from build123d import *

# Parameters (mm, degrees)
SKETCH_1_W          = 29
SKETCH_1_H          = 18
SKETCH_1_R          = 5.5
SKETCH_1_R_2        = 1.5
EXTRUDE_1_DEPTH     = 6
EXTRUDE_2_DEPTH     = 3
SKETCH_2_W          = 3
SKETCH_2_H          = 6
EXTRUDE_3_DEPTH     = 6
SKETCH_4_R          = 1.5
CUT_EXTRUDE_1_DEPTH = 6
SKETCH_5_W          = 3
SKETCH_5_H          = 6
EXTRUDE_4_DEPTH     = 6
SKETCH_7_R          = 1.5
CUT_EXTRUDE_2_DEPTH = 6
FILLET_1_R          = 2
FILLET_3_R          = 1


with BuildPart() as part:
    # Sketch 1 → Extrude 1 (new body)
    with BuildSketch(Plane(origin=(0, 0, 0), x_dir=(1, 0, 0), z_dir=(0, 1, 0))):
        with Locations((15.4, 42.3)):
            Rectangle(SKETCH_1_W, SKETCH_1_H)
        with Locations(Location((15.4, 42.3, 0), (0, 0, 270))):
            Circle(SKETCH_1_R, mode=Mode.SUBTRACT)
        with Locations(Location((6.45, 42.3, 0), (0, 0, 270))):
            Circle(SKETCH_1_R_2, mode=Mode.SUBTRACT)
        with Locations(Location((24.35, 42.3, 0), (0, 0, 270))):
            Circle(SKETCH_1_R_2, mode=Mode.SUBTRACT)
    extrude(amount=EXTRUDE_1_DEPTH)

    # Sketch 1_6 → Extrude 2 (add)
    with BuildSketch(Plane(origin=(0, 0, 0), x_dir=(1, 0, 0), z_dir=(0, 1, 0))):
        with BuildLine():
            ThreePointArc((15.4, 36.8), (19.289087297, 38.410912703), (20.9, 42.3))
            Line((20.9, 42.3), (19.3, 42.3))
            ThreePointArc((19.3, 42.3), (18.157716447, 39.542283553), (15.4, 38.4))
            Line((15.4, 38.4), (15.4, 36.8))
        make_face()
        with BuildLine():
            Line((19.3, 42.3), (20.9, 42.3))
            ThreePointArc((20.9, 42.3), (19.289087297, 46.189087297), (15.4, 47.8))
            Line((15.4, 47.8), (15.4, 46.2))
            ThreePointArc((15.4, 46.2), (18.157716447, 45.057716447), (19.3, 42.3))
        make_face()
        with BuildLine():
            ThreePointArc((9.9, 42.3), (11.510912703, 38.410912703), (15.4, 36.8))
            Line((15.4, 36.8), (15.4, 38.4))
            ThreePointArc((15.4, 38.4), (12.642283553, 39.542283553), (11.5, 42.3))
            Line((11.5, 42.3), (9.9, 42.3))
        make_face()
        with BuildLine():
            Line((15.4, 46.2), (15.4, 47.8))
            ThreePointArc((15.4, 47.8), (11.510912703, 46.189087297), (9.9, 42.3))
            Line((9.9, 42.3), (11.5, 42.3))
            ThreePointArc((11.5, 42.3), (12.642283553, 45.057716447), (15.4, 46.2))
        make_face()
    extrude(amount=EXTRUDE_2_DEPTH)

    # Sketch 2 → Extrude 3 (add)
    with BuildSketch(Plane.ZY.offset(-0.9)):
        with Locations((-46.8, 3)):
            Rectangle(SKETCH_2_W, SKETCH_2_H)
    extrude(amount=EXTRUDE_3_DEPTH)

    # Sketch 4 → Cut-Extrude 1 (cut)
    with BuildSketch(Plane.XY.offset(-45.3)):
        with Locations((-2.1, 3)):
            Circle(SKETCH_4_R)
    extrude(amount=-CUT_EXTRUDE_1_DEPTH, mode=Mode.SUBTRACT)

    # Sketch 5 → Extrude 4 (add)
    with BuildSketch(Plane(origin=(29.9, 0, 0), x_dir=(0, 0, -1), z_dir=(1, 0, 0))):
        with Locations((46.8, 3)):
            Rectangle(SKETCH_5_W, SKETCH_5_H)
    extrude(amount=EXTRUDE_4_DEPTH)

    # Sketch 7 → Cut-Extrude 2 (cut)
    with BuildSketch(Plane(origin=(0, 0, -48.3), x_dir=(-1, 0, 0), z_dir=(0, 0, -1))):
        with Locations((-32.9, 3)):
            Circle(SKETCH_7_R)
    extrude(amount=-CUT_EXTRUDE_2_DEPTH, mode=Mode.SUBTRACT)

    # Fillet 1
    fillet_1_edges = [part.edges().sort_by_distance(p)[0] for p in [
        (29.9, 3, -33.3),
        (0.9, 3, -33.3),
        (0.9, 3, -51.3),
        (29.9, 3, -51.3),
    ]]
    fillet(fillet_1_edges, radius=FILLET_1_R)

    # Fillet 3
    fillet_3_edges = [part.edges().sort_by_distance(p)[0] for p in [
        (-5.1, 0, -46.8),
        (-5.1, 6, -46.8),
        (35.9, 6, -46.8),
        (35.9, 0, -46.8),
    ]]
    fillet(fillet_3_edges, radius=FILLET_3_R)


solid = part.part
The listing builds one solid part. Answer for the finished solid, in the listing's coordinates (mm). A direction names the side the tool comes from. Give positions to 0.01 mm unless a question says otherwise; leave off trailing zeros. Loops run counter-clockwise (first coordinate to the right, second up) from the corner with the lowest first, then second, coordinate; pieces in that order, holes last. Notation, with made-up numbers: (-14.5, 11.5) - (16.5, 11.5) arc R17 ccw to (16.5, 37.5) - close; hole circle Ø4 at (65, 87.5). An arc over 180 degrees is marked (long way). Use one line per item in the form item = value.
1. Section B-B on y = 2.35 is taken. Give the vertices of the cut face in (x, z), then the cut area to 3 significant figures.
Calculated:
outline = (-5.1, -48.3) - (-3.45, -48.3) - (-3.45, -45.3) - (-5.1, -45.3) - close; (-0.75, -48.3) - (0.9, -48.3) - (0.9, -49.3) arc R2 ccw to (2.9, -51.3) - (27.9, -51.3) arc R2 ccw to (29.9, -49.3) - (29.9, -48.3) - (31.55, -48.3) - (31.55, -45.3) - (29.9, -45.3) - (29.9, -35.3) arc R2 ccw to (27.9, -33.3) - (2.9, -33.3) arc R2 ccw to (0.9, -35.3) - (0.9, -45.3) - (-0.75, -45.3) - close; (34.25, -48.3) - (35.9, -48.3) - (35.9, -45.3) - (34.25, -45.3) - close; hole circle Ø3 at (6.45, -42.3); hole circle Ø7.8 at (15.4, -42.3); hole circle Ø3 at (24.35, -42.3)
area = 476 mm^2
2. Which of the six approach directions +Z, -Z, +X, -X, +Y, -Y give full straight-line access (tool end or side, diameter ignored) to faces 5 (the face through (29.9, 3, -49)), 6 (the face through (-0.7, 1.6, -45.3)), 7 (the face through (29.9, 3, -40))?
Calculated:
face_5 = -Z, +X, +Y, -Y
face_6 = +Z, -X, +Y, -Y
face_7 = +Z, +X, +Y, -Y
3. Section C-C on z = -40 is taken. Give the vertices of the cut face in (x, y), then the cut area to 3 significant figures.
Calculated:
outline = (0.9, 0) - (12.25, 0) - (12.25, 3) - (10.4, 3) - (10.4, 6) - (0.9, 6) - close; (18.55, 0) - (29.9, 0) - (29.9, 6) - (20.4, 6) - (20.4, 3) - (18.55, 3) - close
area = 125 mm^2
4. Section D-D on x = 6.45 is taken. Give the vertices of the cut face in (y, z), then the cut area to 3 significant figures.
Calculated:
outline = (0, -51.3) - (6, -51.3) - (6, -43.8) - (0, -43.8) - close; (0, -40.8) - (6, -40.8) - (6, -33.3) - (0, -33.3) - close
area = 90.0 mm^2
5. Given pin 1 Ø0.8 at (y, z) = (2, -49) entering from -X; pin 2 Ø3 at (y, z) = (3.5, -39) entering from +X; pin 3 Ø9 at (x, z) = (15.4, -42.3) entering from +Y, each flat-ended and moving along its own axis, determine where each tip first touches the part or whether it passes through.
Calculated:
pin_1 = 0.9
pin_2 = 29.9
pin_3 = 3
6. The mould has two halves that part along Z. Classify faces 1 (the face through (31.5, 1.6, -48.3)), 2 (the face through (35.599, 0.285, -46.821)), 3 (the face through (13.29, 4.48, -37.22)), 4 (the face through (29.3, 3.04, -33.87)): pulls with the +Z half, pulls with the -Z half, needs draft (parallel to the pull), parting line crosses it, or undercut.
Calculated:
face_1 = pulls with the -Z half
face_2 = needs draft
face_3 = undercut
face_4 = pulls with the +Z half
7. Section A-A on x = 32.9 is taken. Give the vertices of the cut face in (y, z), then the cut area to 3 significant figures.
Calculated:
outline = (0, -48.3) - (1.5, -48.3) - (1.5, -45.3) - (0, -45.3) - close; (4.5, -48.3) - (6, -48.3) - (6, -45.3) - (4.5, -45.3) - close
area = 9.00 mm^2
8. Find the intervals of material crossed by line 1 along X through (y, z) = (4.1, -42.3); line 2 along Y through (x, z) = (-2.1, -47.15); line 3 along X through (y, z) = (1.85, -42.3), in increasing order. Write a range as [from, to].
Calculated:
line_1 = [0.9, 4.95], [7.95, 9.9], [20.9, 22.85], [25.85, 29.9]
line_2 = [0, 1.5], [4.5, 6]
line_3 = [0.9, 4.95], [7.95, 11.5], [19.3, 22.85], [25.85, 29.9]
